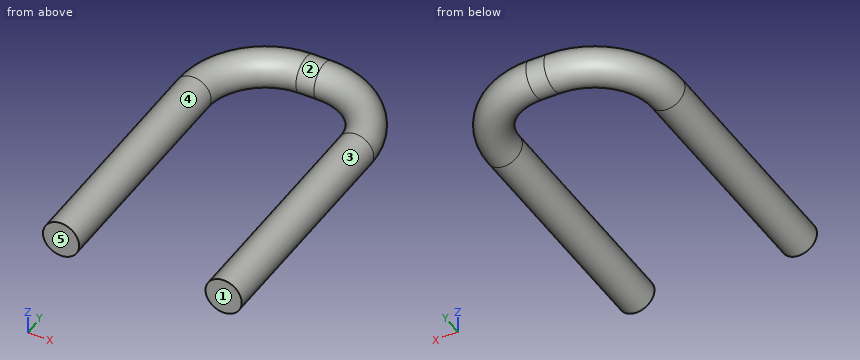
from build123d import *

# Parameters (mm, degrees)
BALAYAGE1_PROFILE_R = 1


with BuildPart() as part:
    # Balayage1: sweep along a path in Esquisse1
    with BuildLine(Plane.XY) as balayage1_path:
        Line((-4.5, 0), (-4.5, 13))
        ThreePointArc((-4.5, 13), (-3.328427125, 15.828427125), (-0.5, 17))
        Line((-0.5, 17), (0.5, 17))
        ThreePointArc((0.5, 17), (3.328427125, 15.828427125), (4.5, 13))
        Line((4.5, 13), (4.5, 0))
    # Balayage1 profile (on start of the path) → Balayage1 (sweep)
    with BuildSketch(Plane(origin=(-4.5, 0, 0), x_dir=(1, 0, 0), z_dir=(0, 1, 0))):
        Circle(BALAYAGE1_PROFILE_R)
    sweep(path=balayage1_path.line)


solid = part.part
Verification items for the finished model (mm, model axes). Face numbers are marked on the shaded views. A direction names the side the tool comes from. Coordinates: 2 decimals unless noted, no trailing zeros. Write each loop counter-clockwise with the first axis right and the second up, starting at its lowest first coordinate (ties: lowest second). Pieces come first, ordered by that corner, then holes. Notation, with made-up numbers: M 0.25,-26 L 33.25,-26 A10 cw 33.25,-19 Z; hole C 3,31.25 d8. An arc over 180 degrees is marked long. Use a Markdown table: item, result.
Q1. Sectioned sample at A-A, the plane y = 4.5. Record the boundary of the cut face in (x, z).
Reply:
| item | result |
|---|---|
| outline | C -4.5,0 d2; C 4.5,0 d2 |
Q2. Sectioned sample at B-B, the plane z = 0. Record the boundary of the cut face in (x, y).
Reply:
| item | result |
|---|---|
| outline | M -5.5,0 L -3.5,0 L -3.5,13 A3 cw -0.5,16 L 0.5,16 A3 cw 3.5,13 L 3.5,0 L 5.5,0 L 5.5,13 A5 ccw 0.5,18 L -0.5,18 A5 ccw -5.5,13 Z |
Q3. Go/stop test with a flat-tipped pin: P1, Ø1.5, axis at x = 1.5, y = 15.5, coming from the -Z side. Record where the tip stops, or that it passes through.
Reply:
| item | result |
|---|---|
| P1 | stops at z = -0.83 |
Q4. Set-up check for the marked faces 1 and 2: record each of +Z, -Z, +X, -X, +Y, -Y from which the full face is reachable in a straight line by a thin tool's end or side.
Reply:
| item | result |
|---|---|
| face 1 | +Z, -Z, +X, -X, -Y |
| face 2 | none |
Q5. Draft check along X on the marked faces 3, 4 and 5. Enter one of: +X half, -X half, draft (parallel to the pull), parting line (faces both ways), or undercut.
Reply:
| item | result |
|---|---|
| face 3 | undercut |
| face 4 | undercut |
| face 5 | draft |
Q6. Thickness scan on line 1 (X direction, y = 2, z = 0.1); line 2 (X direction, y = 3, z = 0.9); line 3 (Z direction, x = 1.5, y = 16.25). Record the ranges inside material, lowest first.
Reply:
| item | result |
|---|---|
| line 1 | x = -5.49 to -3.51, 3.51 to 5.49 |
| line 2 | x = -4.94 to -4.06, 4.06 to 4.94 |
| line 3 | z = -0.8 to 0.8 |
